Autodesk Inventor part; units mm, degrees
ref_plane "Work Plane1" through (66.6877, 0, 0) normal (0, 0, -1) x (1, 0, 0)
ref_plane "YZ Plane" through (0, 0, 0) normal (1, 0, 0) x (0, 1, 0)
ref_plane "XZ Plane" through (0, 0, 0) normal (0, 1, 0) x (-1, 0, 0)
sketch "Sketch1" plane through (0, 0, 0) normal (0, 0, 1) x (1, 0, 0)
  line L0 (15.875, 0) -> (15.875, 1.7526)
  line L1 (15.875, 1.7526) -> (2.4638, 1.7526)
  line L2 (0, 3.3401) -> (0, 1.2192)
  line L3 (0, 1.2192) -> (1.6764, 1.2192)
  line L4 (1.6764, 1.2192) -> (2.3803, 0)
  line L5 (2.3803, 0) -> (15.875, 0)
  line L6 (0, 3.3401) -> (0.6376, 3.3401)
  line L7 (0.6376, 3.3401) -> (2.4638, 1.7526)
  line L8 (-3.175, 0) -> (19.05, 0)
  line L9 (0, -0.668) -> (0, 4.0081)
  dimension "d0" = 15.875
  dimension "d1" = 1.6764
  dimension "d2" = 3.5052
  dimension "d3" = 2.4638
  dimension "d4" = 41
  dimension "d5" = 2.4384
  dimension "d6" = 60
  dimension "d7" = 6.6802
revolve "Body" add sketch "Sketch1" angle 360 about axis through (2.3803, 0, 0) along (1, 0, 0) contours L5 L4 L3 L2 L6 L7 L1 L0
sketch "Sketch2" plane through (0, 0, 0) normal (-1, 0, 0) x (0, 0, 1)
  circle A0 centre (0, 0) radius 3.3401
  circle A1 centre (0, 0) radius 1.2192
  line L0 (0.9421, 0.2524) -> (1.1777, 0.3156)
  line L1 (0.9421, -0.2524) -> (1.1777, -0.3156)
  arc A2 (0.9421, -0.2524) -> (0.9421, 0.2524) centre (0, 0) ccw
  arc A3 (1.1777, -0.3156) -> (1.1777, 0.3156) centre (0, 0) ccw
  line L2 (0, -4.6761) -> (0, 4.6761)
  line L3 (-4.6761, 0) -> (4.6761, 0)
  line L4 (0.9421, 0.2524) -> (0, 0) construction
  line L5 (0, 0) -> (0.9421, -0.2524) construction
  line L6 (0.2524, 0.9421) -> (0.3156, 1.1777)
  line L7 (0.6897, 0.6897) -> (0.8621, 0.8621)
  arc A4 (0.6897, 0.6897) -> (0.2524, 0.9421) centre (0, 0) ccw
  arc A5 (0.8621, 0.8621) -> (0.3156, 1.1777) centre (0, 0) ccw
  line L8 (-0.6897, 0.6897) -> (-0.8621, 0.8621)
  line L9 (-0.2524, 0.9421) -> (-0.3156, 1.1777)
  arc A6 (-0.2524, 0.9421) -> (-0.6897, 0.6897) centre (0, 0) ccw
  arc A7 (-0.3156, 1.1777) -> (-0.8621, 0.8621) centre (0, 0) ccw
  line L10 (-0.9421, -0.2524) -> (-1.1777, -0.3156)
  line L11 (-0.9421, 0.2524) -> (-1.1777, 0.3156)
  arc A8 (-0.9421, 0.2524) -> (-0.9421, -0.2524) centre (0, 0) ccw
  arc A9 (-1.1777, 0.3156) -> (-1.1777, -0.3156) centre (0, 0) ccw
  line L12 (-0.2524, -0.9421) -> (-0.3156, -1.1777)
  line L13 (-0.6897, -0.6897) -> (-0.8621, -0.8621)
  arc A10 (-0.6897, -0.6897) -> (-0.2524, -0.9421) centre (0, 0) ccw
  arc A11 (-0.8621, -0.8621) -> (-0.3156, -1.1777) centre (0, 0) ccw
  line L14 (0.6897, -0.6897) -> (0.8621, -0.8621)
  line L15 (0.2524, -0.9421) -> (0.3156, -1.1777)
  arc A12 (0.2524, -0.9421) -> (0.6897, -0.6897) centre (0, 0) ccw
  arc A13 (0.3156, -1.1777) -> (0.8621, -0.8621) centre (0, 0) ccw
  dimension "d8" = 1.9507
  dimension "d9" = 2.4384
  dimension "d10" = 15
  dimension "d11" = 15
  dimension "d22" = 360
extrude "Slot" add sketch "Sketch2" against normal up to next contours L3 A2 L0 A1 | A1 L1 A2 L3 | L3 A8 L10 A1 | A1 L11 A8 L3 | A1 L7 A4 L6 | L9 A6 L8 A1 | A1 L13 A10 L12 | L15 A12 L14 A1
thread "Thread"
chamfer "Chamfer1" distance 0.4724 distance2 0.9449 1 edges at (15.875, -1.7526, 0) measured on face at (15.875, -0.7696, -0.2093)
ref_plane "Work Plane1" through (66.6877, 0, 0) normal (0, 0, -1) x (1, 0, 0)
equation "\"d0\" = NLG"
equation "\"d1\" = INTI"
equation "\"d2\" = GD"
equation "\"d3\" = KOH"
equation "\"d4\" = 0.5 * SEWI"
equation "\"d5\" = SW"
equation "\"d7\" = KOD"
equation "\"d8\" = 0.8 * SW"
equation "\"d9\" = SW"
equation "\"d15\" = GEL"
equation "\"d17\" = -0.5 * SPD + 0.5 * GD"
equation "\"d18\" = GUL"
equation "\"NLG\" = 15.875"
equation "\"SW\" = 2.4384"
equation "\"INTI\" = 1.6764"
equation "\"GEL\" = 11.42695"
equation "\"KOH\" = 2.4638"
equation "\"KOD\" = 6.6802"
equation "\"GUL\" = 0.94488"
equation "\"SPD\" = 2.56032"
equation "\"GD\" = NND"
equation "\"SEWI\" = 82deg"
equation "\"TOA\" = 30deg"
equation "\"GD1\" = SPD"
equation "\"EPV\" = 4.4794"
equation "\"THREADDIA\" = 3.5052"
equation "\"BDM\" = NND"
equation "\"NND\" = 3.5052"
equation "\"GAL\" = 1.9845"
equation "\"E0\" = 1.155 * SW"
properties part number "ANSI B18.3 - 6-32 UNC x 0.625, SSFCHCSI" material "Steel, Mild"
Can you work these out from the model? Positions are in its coordinate system, mm. A direction names the side the tool comes from. Coordinates: 2 decimals unless noted, no trailing zeros. Loops run counter-clockwise (first coordinate to the right, second up) from the corner with the lowest first, then second, coordinate; pieces in that order, holes last. Notation, with made-up numbers: (-28, 78) - (-23, 78) arc R7 cw to (-23, 84) - close; hole circle Ø1 at (46, -4). An arc over 180 degrees is marked (long way). Put each result on its own line as item: value. Start each with the question number.
Item 1: If we mould it in two halves opening along Y, with no side actions, what happens to faces 1 (the face through (15.875, 0, 0)), 2 (the face through (2.35, -0.4, 1.81)), 3 (the face through (2.34, -0.02, 0.07))? For each: +Y half, -Y half, draft (parallel to the pull), parting line (faces both ways), or undercut.
Item 2: If I drill on line 1 along Y through (x, z) = (1.5, -0.75); line 2 along Z through (x, y) = (6.25, 0.5); line 3 along X through (y, z) = (-0.5, 1.5), over which ranges is the centre line in solid material (lowest first)?
Item 3: For pin 1 (1 mm diameter, centred on x = 5.5, y = -0.5, fed in from -Z); pin 2 (3 mm diameter, centred on x = 12.5, z = -1, fed in from -Y); pin 3 (1 mm diameter, centred on y = -2, z = 0, fed in from +X), each with a flat end and sliding along its axis, tell me the tip position at first contact or that it passes through.
Item 4: Suppose I cut it at A-A (x = 11.25). Please give me the cut outline in (y, z).
Item 5: Which directions (+Z, -Z, +X, -X, +Y, -Y) give clear straight access to the entire face, cutting with the end or side of a thin tool? Please do faces 4 (the face through (0, -1, -1)), 5 (the face through (8.61, 1.67, -0.53)).
Here are the results:
1. face 1: draft
1. face 2: parting line
1. face 3: undercut
2. line 1: -2.48 to -0.75, 0.75 to 2.48
2. line 2: -1.68 to 1.68
2. line 3: 0 to 15.27
3. pin 1: z = -1.75
3. pin 2: y = -1.75
3. pin 3: x = 15.44
4. outline: circle Ø3.51 at (0, 0)
5. face 4: +Z, -Z, -X, +Y, -Y
5. face 5: +X
